```python
from build123d import *

# Parameters (mm, degrees)
SKETCH1_W           = 146.4
SKETCH1_H           = 95.25
BOSS_EXTRUDE1_DEPTH = 3
SKETCH2_W           = 6
SKETCH2_H           = 12.7
BOSS_EXTRUDE2_DEPTH = 6
SKETCH3_W           = 12.7
SKETCH3_H           = 6
CUT_EXTRUDE1_DEPTH  = 93.610909859
LPATTERN3_COUNT     = 3
LPATTERN3_PITCH     = 25.4
LPATTERN3_COL_COUNT = 3
LPATTERN3_COL_PITCH = 25.4
CUT_EXTRUDE2_DEPTH  = 93.610909859
FILLET1_R           = 2.54


with BuildPart() as part:
    # Sketch1 → Boss-Extrude1 (new, symmetric)
    with BuildSketch(Plane(origin=(0, 0, 0), x_dir=(1, 0, 0), z_dir=(0, 1, 0))):
        Rectangle(SKETCH1_W, SKETCH1_H)
    extrude(amount=BOSS_EXTRUDE1_DEPTH, both=True)

    # Sketch2 → Boss-Extrude2 (add)
    with BuildSketch(Plane(origin=(0, 3, 0), x_dir=(1, 0, 0), z_dir=(0, 1, 0))):
        with Locations((-76.2, 38.1)):
            Rectangle(SKETCH2_W, SKETCH2_H)
        with Locations((-76.2, -38.1)):
            Rectangle(SKETCH2_W, SKETCH2_H)
    boss_extrude2 = extrude(amount=-BOSS_EXTRUDE2_DEPTH)

    # Mirror1: Boss-Extrude2 across plane
    add(boss_extrude2.mirror(Plane(origin=(0, 0, 0), x_dir=(0, 0, 1), z_dir=(1, 0, 0))))

    # Sketch3 → Cut-Extrude1 (cut, symmetric)
    with BuildSketch(Plane(origin=(0, 3, 0), x_dir=(1, 0, 0), z_dir=(0, 1, 0))):
        with Locations((0, -40.005)):
            Rectangle(SKETCH3_W, SKETCH3_H)
        with Locations((0, 40.005)):
            Rectangle(SKETCH3_W, SKETCH3_H)
    cut_extrude1 = extrude(amount=CUT_EXTRUDE1_DEPTH, both=True, mode=Mode.SUBTRACT)

    # LPattern3: Cut-Extrude1 ×3
    with Locations(*[(i * LPATTERN3_PITCH, 0, 0) for i in range(1, LPATTERN3_COUNT)]):
        add(cut_extrude1, mode=Mode.SUBTRACT)

    # LPattern3 col: Cut-Extrude1 ×3
    with Locations(*[(-i * LPATTERN3_COL_PITCH, 0, 0) for i in range(1, LPATTERN3_COL_COUNT)]):
        add(cut_extrude1, mode=Mode.SUBTRACT)

    # Sketch4 → Cut-Extrude2 (cut, through all)
    with BuildSketch(Plane(origin=(0, 3, 0), x_dir=(1, 0, 0), z_dir=(0, 1, 0))):
        Polygon((-3.175, 30.655), (-59.232948188, 30.655), (-3.175, 4.948845898), align=None)
        Polygon((-7.617051812, 0), (-66.85, 27.16209464), (-66.85, -27.16209464), align=None)
        Polygon((-3.175, -4.948845898), (-59.232948188, -30.655), (-3.175, -30.655), align=None)
        Polygon((59.232948188, -30.655), (3.175, -4.948845898), (3.175, -30.655), align=None)
        Polygon((66.85, 27.16209464), (7.617051812, 0), (66.85, -27.16209464), align=None)
        Polygon((59.232948188, 30.655), (3.175, 30.655), (3.175, 4.948845898), align=None)
    extrude(amount=-CUT_EXTRUDE2_DEPTH, mode=Mode.SUBTRACT)

    # Fillet1
    fillet1_edges = [part.edges().sort_by_distance(p)[0] for p in [
        (-3.175, 0, 4.948845898),
        (-3.175, 0, 30.655),
        (-59.232948188, 0, 30.655),
        (-7.617051812, 0, 0),
        (-66.85, 0, 27.16209464),
        (-66.85, 0, -27.16209464),
        (66.85, 0, -27.16209464),
        (66.85, 0, 27.16209464),
        (7.617051812, 0, 0),
        (3.175, 0, 4.948845898),
        (59.232948188, 0, 30.655),
        (3.175, 0, 30.655),
        (3.175, 0, -30.655),
        (59.232948188, 0, -30.655),
        (3.175, 0, -4.948845898),
        (-59.232948188, 0, -30.655),
        (-3.175, 0, -30.655),
        (-3.175, 0, -4.948845898),
        (-73.2, 0, -47.625),
        (73.2, 0, -47.625),
        (73.2, 0, 47.625),
        (-73.2, 0, 47.625),
    ]]
    fillet(fillet1_edges, radius=FILLET1_R)


solid = part.part
```
Input: part model. Units: mm. Frame: model coordinates. A direction names the side the tool comes from. Coordinates: 2 decimals unless noted, no trailing zeros. Write each loop counter-clockwise with the first axis right and the second up, starting at its lowest first coordinate (ties: lowest second). Pieces come first, ordered by that corner, then holes.
1) Mould query, pull axis X, two halves, no side actions, for faces 1 (the flat face through (25, 0, 37.005)), 2 (the flat face through (76, 0, -44.45)), 3 (the flat face through (79.2, 0, -38)). Classes: pulls with the +X half, pulls with the -X half, needs draft (parallel to the pull), parting line crosses it, or undercut.
2) Section C-C on z = 13.5. Output: boundary loops of the cut face in (x, y) (3 decimals).
3) Set-up query: faces 4 (the flat face through (-76, 0, -31.75)), 5 (the flat face through (19.05, 0, 40)), 6 (the flat face through (76, 0, 31.75)). Return all of +Z, -Z, +X, -X, +Y, -Y with unobstructed straight access to the full face (end or side cutting, diameter ignored); none if empty.
4) Section B-B on x = 42. Output: boundary loops of the cut face in (y, z) (3 decimals).
5) Section D-D on y = 2. State how many separate pieces and enclosed holes the cut face has, and give its area (3 significant figures).
6) Pin query (flat end, axial travel): pin 1 Ø1 at (y, z) = (1.5, -19) entering from +X; pin 2 Ø3 at (x, y) = (-77.5, 0) entering from -Z; pin 3 Ø1.8 at (x, y) = (-76.5, -0.5) entering from +Z. Return the tip coordinate at first contact, or that it passes through.
7) Section A-A on z = 39.5. Output: boundary loops of the cut face in (x, y).
8) Material intervals for line 1 along X through (y, z) = (-2.5, -38); line 2 along Z through (x, y) = (3, 2) (3 decimals); line 3 along X through (y, z) = (-0.25, 15) (3 decimals), sorted ascending.
Check result:
1. face 1: undercut
1. face 2: needs draft
1. face 3: pulls with the +X half
2. outline: (-73.2, -3) - (-66.85, -3) - (-66.85, 3) - (-73.2, 3) - close; (-37.057, -3) - (-21.823, -3) - (-21.823, 3) - (-37.057, 3) - close; (-3.175, -3) - (3.175, -3) - (3.175, 3) - (-3.175, 3) - close; (21.823, -3) - (37.057, -3) - (37.057, 3) - (21.823, 3) - close; (66.85, -3) - (73.2, -3) - (73.2, 3) - (66.85, 3) - close
3. face 4: -X, +Y, -Y
3. face 5: +Y, -Y
3. face 6: +X, +Y, -Y
4. outline: (-3, -47.625) - (3, -47.625) - (3, -30.655) - (-3, -30.655) - close; (-3, -22.753) - (3, -22.753) - (3, -15.767) - (-3, -15.767) - close; (-3, 15.767) - (3, 15.767) - (3, 22.753) - (-3, 22.753) - close; (-3, 30.655) - (3, 30.655) - (3, 47.625) - (-3, 47.625) - close
5. separate pieces: 1
5. enclosed holes: 16
5. area: 7,510 mm2
6. pin 1: stops at x = 73.2
6. pin 2: stops at z = -44.45
6. pin 3: stops at z = 44.45
7. outline: (-79.2, -3) - (-57.15, -3) - (-57.15, 3) - (-79.2, 3) - close; (-44.45, -3) - (-31.75, -3) - (-31.75, 3) - (-44.45, 3) - close; (-19.05, -3) - (-6.35, -3) - (-6.35, 3) - (-19.05, 3) - close; (6.35, -3) - (19.05, -3) - (19.05, 3) - (6.35, 3) - close; (31.75, -3) - (44.45, -3) - (44.45, 3) - (31.75, 3) - close; (57.15, -3) - (79.2, -3) - (79.2, 3) - (57.15, 3) - close
8. line 1: x = -79.2 to -57.15, -44.45 to -31.75, -19.05 to -6.35, 6.35 to 19.05, 31.75 to 44.45, 57.15 to 79.2
8. line 2: z = -47.625 to -43.005, -37.005 to 37.005, 43.005 to 47.625
8. line 3: x = -73.2 to -66.85, -40.328 to -25.094, -3.175 to 3.175, 25.094 to 40.328, 66.85 to 73.2
